Part model, mm, in its own coordinate system. A direction names the side the tool comes from. Give positions to 0.01 mm unless a question says otherwise; leave off trailing zeros. Order: outer loops, then holes, each group sorted by start corner. A loop starts at its lowest first (then second) coordinate and runs counter-clockwise, first axis right, second up. Notation, with made-up numbers: M 20,-39 L 30,-39 A24 cw 30,-29 Z; hole C 19,44 d11. An arc over 180 degrees is marked long. Answer as a JSON object with one key per item and string values.
from build123d import *

# Parameters (mm, degrees)
SKETCH1_W               = 120
SKETCH1_H               = 180
BOSS_EXTRUDE1_DEPTH     = 5
SKETCH3_W               = 40
SKETCH3_H               = 20
CUT_EXTRUDE2_DEPTH      = 5
MIRROR2_COPY_1_SKETCH_W = 40
MIRROR2_COPY_1_SKETCH_H = 20
MIRROR2_COPY_1_DEPTH    = 5


with BuildPart() as part:
    # Sketch1 → Boss-Extrude1 (new body)
    with BuildSketch(Plane(origin=(0, 0, 0), x_dir=(1, 0, 0), z_dir=(0, 1, 0))):
        with Locations((60, 90)):
            Rectangle(SKETCH1_W, SKETCH1_H)
    extrude(amount=BOSS_EXTRUDE1_DEPTH)

    # Sketch3 → Cut-Extrude2 (cut)
    with BuildSketch(Plane.XZ):
        with Locations((30, -160)):
            Rectangle(SKETCH3_W, SKETCH3_H)
    cut_extrude2 = extrude(amount=-CUT_EXTRUDE2_DEPTH, mode=Mode.SUBTRACT)

    # Mirror1: Cut-Extrude2 across plane
    add(cut_extrude2.mirror(Plane.ZY.offset(-60)), mode=Mode.SUBTRACT)

    # Mirror2: Cut-Extrude2 across plane
    add(cut_extrude2.mirror(Plane(origin=(0, 0, -90), x_dir=(1, 0, 0), z_dir=(0, 0, -1))), mode=Mode.SUBTRACT)

    # Mirror2 copy 1 sketch → Mirror2 copy 1 (cut)
    with BuildSketch(Plane(origin=(120, 0, -180), x_dir=(-1, 0, 0), z_dir=(0, -1, 0))):
        with Locations((30, -160)):
            Rectangle(MIRROR2_COPY_1_SKETCH_W, MIRROR2_COPY_1_SKETCH_H)
    extrude(amount=-MIRROR2_COPY_1_DEPTH, mode=Mode.SUBTRACT)


solid = part.part
1. Cut at B-B on z = -166. Give the cut face in (x, y).
Worked answers:
{"outline": "M 0,0 L 10,0 L 10,5 L 0,5 Z; M 50,0 L 70,0 L 70,5 L 50,5 Z; M 110,0 L 120,0 L 120,5 L 110,5 Z"}
2. Which spindle directions (+Z, -Z, +X, -X, +Y, -Y) get a long thin tool onto all of the face, cutting with end or side? Do faces 1 (the flat face through (59, 5, -91)), 2 (the flat face through (50, 2, -160)). Say none if no direction does.
Worked answers:
{"face 1": "+Z, -Z, +X, -X, +Y", "face 2": "+Y, -Y"}
3. Pin check, flat tip, straight feed: P1, Ø2, axis at x = 40, z = -28.5, coming from the -Y side. Stop position of the tip, or through.
Worked answers:
{"P1": "passes through"}
4. Cut at A-A on x = 24. Give the cut face in (y, z), plus the area to 3 significant figures.
Worked answers:
{"outline": "M 0,-180 L 5,-180 L 5,-170 L 0,-170 Z; M 0,-150 L 5,-150 L 5,-30 L 0,-30 Z; M 0,-10 L 5,-10 L 5,0 L 0,0 Z", "area": "700 mm^2"}
5. Cut at C-C on y = 3.1. Give the cut face in (x, z), plus the area to 3 significant figures.
Worked answers:
{"outline": "M 0,-180 L 120,-180 L 120,0 L 0,0 Z; hole M 10,-170 L 50,-170 L 50,-150 L 10,-150 Z; hole M 10,-30 L 50,-30 L 50,-10 L 10,-10 Z; hole M 70,-170 L 110,-170 L 110,-150 L 70,-150 Z; hole M 70,-30 L 110,-30 L 110,-10 L 70,-10 Z", "area": "18,400 mm^2"}
6. Probe line 1 along Z through (x, y) = (94, 2.1); line 2 along X through (y, z) = (4.85, -26). List the from-to ranges inside material, lowest first.
Worked answers:
{"line 1": "z = -180 to -170, -150 to -30, -10 to 0", "line 2": "x = 0 to 10, 50 to 70, 110 to 120"}
7. Two-plate mould, pull along Z, no slides. Class faces 3 (the flat face through (59, 2, 0)), 4 (the flat face through (110, 2, -20)), 5 (the flat face through (59, 2, -180)), 6 (the flat face through (0, 2, -89)): +Z half, -Z half, draft (parallel to the pull), parting line (faces both ways), or undercut.
Worked answers:
{"face 3": "+Z half", "face 4": "undercut", "face 5": "-Z half", "face 6": "draft"}
